from build123d import *

# Parameters (mm, degrees)
F0_R      = 15
F1_DEPTH  = 35
F2_R      = 5
F3_DEPTH  = 35.001
F4_R      = 5.5
F5_DEPTH  = 12.5
F6_W      = 1.5
F6_H      = 20
F7_DEPTH  = 35.001
F8_R      = 1.45
F9_DEPTH  = 12.5
F11_R     = 2.9
F12_DEPTH = 10
F14_R     = 2.9
F15_DEPTH = 10
F16_SIZE  = 1.5


with BuildPart() as f1:
    # F0 (on Top) → F1 (new body)
    with BuildSketch(Plane.XY):
        Circle(F0_R)
    extrude(amount=F1_DEPTH)

    # F2 (on face) → F3 (cut, through all)
    with BuildSketch(Plane.XY.offset(35)):
        Circle(F2_R)
    extrude(amount=-F3_DEPTH, mode=Mode.SUBTRACT)

    # F4 (on face) → F5 (cut)
    with BuildSketch(Plane(origin=(0, 0, 0), x_dir=(1, 0, 0), z_dir=(0, 0, -1))):
        Circle(F4_R)
    extrude(amount=-F5_DEPTH, mode=Mode.SUBTRACT)

    # F6 (on face) → F7 (cut, through all)
    with BuildSketch(Plane(origin=(0, 0, 0), x_dir=(1, 0, 0), z_dir=(0, 0, -1))):
        with Locations((0, -10)):
            Rectangle(F6_W, F6_H)
    extrude(amount=-F7_DEPTH, mode=Mode.SUBTRACT)

    # F8 (on Right) → F9 (cut, symmetric)
    with BuildSketch(Plane.YZ):
        with Locations((10, 5.5)):
            Circle(F8_R)
        with Locations((10, 29.5)):
            Circle(F8_R)
    extrude(amount=F9_DEPTH, both=True, mode=Mode.SUBTRACT)

    # F11 (on offset) → F12 (cut)
    with BuildSketch(Plane.YZ.offset(15)):
        with Locations((10, 5.5)):
            Circle(F11_R)
    extrude(amount=-F12_DEPTH, mode=Mode.SUBTRACT)

    # F14 (on offset) → F15 (cut)
    with BuildSketch(Plane.YZ.offset(-15)):
        with Locations((10, 29.5)):
            Circle(F14_R)
    extrude(amount=F15_DEPTH, mode=Mode.SUBTRACT)

    # F16
    f16_edges = [f1.edges().sort_by_distance(p)[0] for p in [
        (-10.338037, -10.868533, 0),
        (-10.338037, -10.868533, 35),
    ]]
    chamfer(f16_edges, length=F16_SIZE)


solid = f1.part
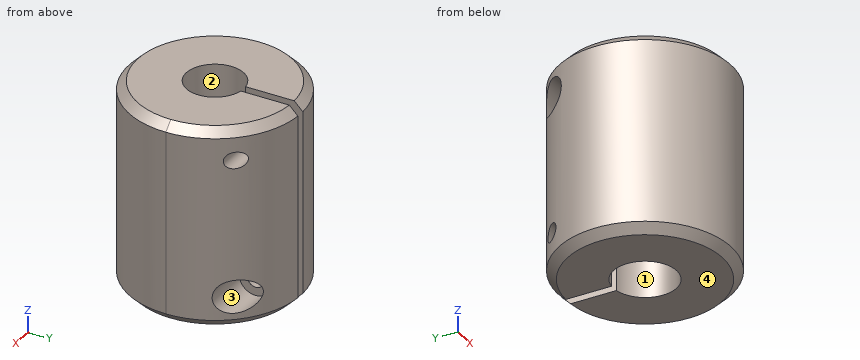
Geometry: final body of the model. Coordinates: model frame, mm. Face numbers are marked on the shaded views. A direction names the side the tool comes from. Round coordinates to 2 decimals unless told otherwise and drop trailing zeros. Loops run counter-clockwise (first coordinate to the right, second up) from the corner with the lowest first, then second, coordinate; pieces in that order, holes last. Notation, with made-up numbers: M -29,-19.5 L 20,-19.5 A15 ccw 20,8.5 Z; hole C 80.5,43.5 d1. An arc over 180 degrees is marked long. One line per question, with ' | ' between items.
(1) Material intervals for line 1 along Z through (x, y) = (9, 10); line 2 along Z through (x, y) = (-8.5, 10); line 3 along X through (y, z) = (0, 5.25), sorted ascending. Write a range as from..to.
Check result:
line 1: z = 0..2.6, 8.4..28.05, 30.95..35 | line 2: z = 0..4.05, 6.95..26.6, 32.4..35 | line 3: x = -15..-5.5, 5.5..15
(2) Cut plane A-A on x = 0. Return the cut outline in (y, z).
Check result:
outline: M -15,1.5 L -13.5,0 L -5.5,0 L -5.5,12.5 L -5,12.5 L -5,35 L -13.5,35 L -15,33.5 Z
(3) Cut plane C-C on z = 19. Return the cut outline in (x, y).
Check result:
outline: M -0.75,4.94 L -0.75,14.98 A15 ccw long 0.75,14.98 L 0.75,4.94 A5 cw long Z
(4) Pull-direction query (Y, two-part tool) for the marked faces 3 and 4; classes: +Y half, -Y half, draft (parallel to the pull), parting line (faces both ways), or undercut.
Check result:
face 3: undercut | face 4: draft
(5) Cut plane D-D on y = 10. Give the number of separate pieces and of enclosed holes in the cut face, plus the area to 3 significant figures.
Check result:
separate pieces: 6 | enclosed holes: 0 | area: 567 mm2
(6) Access query for the marked faces 1 and 2. Directions: +Z, -Z, +X, -X, +Y, -Y. A direction counts if a zero-diameter tool reaches every point of the face in a straight line with its end or side. Return the directions, or none.
Check result:
face 1: -Z | face 2: +Z, -Z
(7) Contact query for flat-ended pins moving along their axis: P1, Ø4.5, axis at y = 10, z = 5.5, coming from the -X side; P2, Ø11, axis at y = 7.5, z = 18.5, coming from the +X side; P3, Ø1.7, axis at y = 10.5, z = 28, coming from the -X side. Output: stop coordinate, or through.
Check result:
P1: stops at x = -12.84 | P2: stops at x = 14.87 | P3: stops at x = -5
(8) Cut plane B-B on z = 5.5. Return the cut outline in (x, y), plus the area to 3 significant figures.
Check result:
outline: M -12.32,8.55 A15 ccw long 13.21,7.1 L 5,7.1 L 5,8.55 L 0.75,8.55 L 0.75,5.45 A5.5 cw long -0.75,5.45 L -0.75,8.55 Z; M -9.69,11.45 L -0.75,11.45 L -0.75,14.98 A15 ccw Z; M 0.75,11.45 L 5,11.45 L 5,12.9 L 7.65,12.9 A15 ccw 0.75,14.98 Z | area: 521 mm2
